The model under review builds one solid part; all positions refer to its coordinate system, in mm. Face numbers are marked on the shaded views. A direction names the side the tool comes from. Coordinates: 2 decimals unless noted, no trailing zeros. Write each loop counter-clockwise with the first axis right and the second up, starting at its lowest first coordinate (ties: lowest second). Pieces come first, ordered by that corner, then holes.
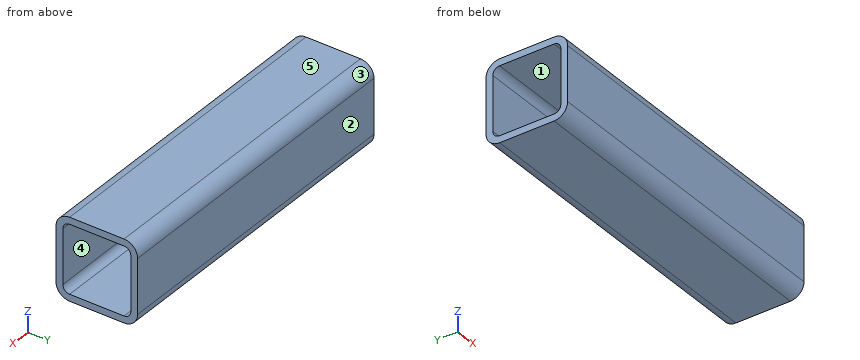
Autodesk Inventor part; units mm, degrees
ref_plane "YZ Plane" through (0, 0, 0) normal (1, 0, 0) x (0, 1, 0)
ref_plane "XZ Plane" through (0, 0, 0) normal (0, 1, 0) x (-1, 0, 0)
ref_plane "XY Plane" through (0, 0, 0) normal (0, 0, 1) x (1, 0, 0)
sketch "Sketch5" plane through (0, 0, 0) normal (1, 0, 0) x (0, 1, 0)
  line L0 (-25.4, 38.1) -> (25.4, 38.1)
  line L1 (38.1, 25.4) -> (38.1, -25.4)
  line L2 (25.4, -38.1) -> (-25.4, -38.1)
  line L3 (-38.1, -25.4) -> (-38.1, 25.4)
  line L4 (-38.1, 38.1) -> (38.1, -38.1) construction
  line L5 (38.1, 38.1) -> (-38.1, -38.1) construction
  arc A0 (38.1, 25.4) -> (25.4, 38.1) centre (25.4, 25.4) ccw
  arc A1 (25.4, -38.1) -> (38.1, -25.4) centre (25.4, -25.4) ccw
  arc A2 (-38.1, -25.4) -> (-25.4, -38.1) centre (-25.4, -25.4) ccw
  arc A3 (-25.4, 38.1) -> (-38.1, 25.4) centre (-25.4, 25.4) ccw
  line L6 (31.75, -25.4) -> (31.75, 25.4)
  arc A4 (31.75, 25.4) -> (25.4, 31.75) centre (25.4, 25.4) ccw
  line L7 (25.4, 31.75) -> (-25.4, 31.75)
  arc A5 (-25.4, 31.75) -> (-31.75, 25.4) centre (-25.4, 25.4) ccw
  line L8 (-31.75, 25.4) -> (-31.75, -25.4)
  arc A6 (-31.75, -25.4) -> (-25.4, -31.75) centre (-25.4, -25.4) ccw
  line L9 (-25.4, -31.75) -> (25.4, -31.75)
  arc A7 (25.4, -31.75) -> (31.75, -25.4) centre (25.4, -25.4) ccw
  point P0 (0, 0)
  dimension "d6" = 76.2
  dimension "d7" = 76.2
  dimension "d8" = 12.7
  dimension "d9" = 6.35
extrude "Extrusion4" add sketch "Sketch5" along normal mid plane 304.8
properties part number "Front Hitch Model-1_Base Tube-3" material "SS304"
Item 1: For pin 1 (6 mm diameter, centred on x = 43.5, y = 29, fed in from -Z), flat-tipped, find the tip position at first contact; note if it passes through.
Solved:
pin 1: stops at z = -38.09
Item 2: Mouldability with a two-part tool opening along Z and no side actions: class the marked faces 1, 2 and 3 as pulls with the +Z half, pulls with the -Z half, needs draft (parallel to the pull), parting line crosses it, or undercut.
Solved:
face 1: undercut
face 2: needs draft
face 3: pulls with the +Z half
Item 3: Take a section at C-C, the plane x = 9. Write out the cut boundary in (y, z), plus the area to 3 significant figures.
Solved:
outline: (-38.1, -25.4) arc R12.7 ccw to (-25.4, -38.1) - (25.4, -38.1) arc R12.7 ccw to (38.1, -25.4) - (38.1, 25.4) arc R12.7 ccw to (25.4, 38.1) - (-25.4, 38.1) arc R12.7 ccw to (-38.1, 25.4) - close; hole (-31.75, -25.4) arc R6.35 ccw to (-25.4, -31.75) - (25.4, -31.75) arc R6.35 ccw to (31.75, -25.4) - (31.75, 25.4) arc R6.35 ccw to (25.4, 31.75) - (-25.4, 31.75) arc R6.35 ccw to (-31.75, 25.4) - close
area: 1,670 mm2
Item 4: Take a section at A-A, the plane z = 10. Write out the cut boundary in (x, y).
Solved:
outline: (-152.4, -38.1) - (152.4, -38.1) - (152.4, -31.75) - (-152.4, -31.75) - close; (-152.4, 31.75) - (152.4, 31.75) - (152.4, 38.1) - (-152.4, 38.1) - close
Item 5: Machinability: for the marked faces 4 and 5, which of the approach directions +Z, -Z, +X, -X, +Y, -Y give a long, thin tool a straight path to every point of the face, cutting with its end or side? Answer none if there is none.
Solved:
face 4: +X, -X
face 5: +Z, +X, -X, +Y, -Y
Item 6: To check wall thickness, follow line 1 along Y through (x, z) = (31.5, -18); line 2 along Y through (x, z) = (-111.5, -28). State the ranges of each line that lie inside material, in increasing order.
Solved:
line 1: y = -38.1 to -31.75, 31.75 to 38.1
line 2: y = -37.83 to -31.19, 31.19 to 37.83
